```python
from build123d import *

# Parameters (mm, degrees)
ESQUISSE1_R             = 1.5
BOSS_EXTRU_1_DEPTH      = 10.4
ESQUISSE2_R             = 1.5
BOSS_EXTRU_3_DEPTH      = 0.2
BOSS_EXTRU_4_START      = 0.2
ESQUISSE3_R             = 1.5
BOSS_EXTRU_4_DEPTH      = 0.2
ENL_V_MAT_EXTRU_1_DEPTH = 0.2
ENL_V_MAT_EXTRU_3_DEPTH = 0.5
ENL_V_MAT_EXTRU_4_DEPTH = 0.5
CONG_1_R                = 0.4
ESQUISSE8_R             = 2
BOSS_EXTRU_5_DEPTH      = 3
CONG_2_R                = 0.4
ESQUISSE9_W             = 7
ESQUISSE9_H             = 12.59732845
ESQUISSE9_R             = 1.25
ENL_V_MAT_EXTRU_5_DEPTH = 0.1
BOSS_EXTRU_6_START      = 0.75
BOSS_EXTRU_6_DEPTH      = 0.75
BOSS_EXTRU_7_START      = 1
BOSS_EXTRU_7_DEPTH      = 1
CONG_3_R                = 1


with BuildPart() as part:
    # Esquisse1 → Boss.-Extru.1 (new body)
    with BuildSketch(Plane(origin=(0, 0, 0), x_dir=(0, 0, -1), z_dir=(1, 0, 0))):
        with BuildLine():
            Line((2.8, 0), (15, 0))
            Line((15, 0), (20, 5))
            Line((20, 5), (20, 31))
            Line((20, 31), (2.8, 31))
            ThreePointArc((2.8, 31), (0.820101013, 30.179898987), (0, 28.2))
            Line((0, 28.2), (0, 2.8))
            ThreePointArc((0, 2.8), (0.820101013, 0.820101013), (2.8, 0))
        make_face()
        with Locations((3, 28.2)):
            Circle(ESQUISSE1_R, mode=Mode.SUBTRACT)
        with Locations((3, 2.8)):
            Circle(ESQUISSE1_R, mode=Mode.SUBTRACT)
    extrude(amount=BOSS_EXTRU_1_DEPTH)

    # Esquisse2 → Boss.-Extru.3 (add)
    with BuildSketch(Plane(origin=(10.4, 0, 0), x_dir=(0, 0, -1), z_dir=(1, 0, 0))):
        with BuildLine():
            Line((5.15, 28.2), (5.15, 2.8))
            ThreePointArc((5.15, 2.8), (3, 0.65), (0.85, 2.8))
            Line((0.85, 2.8), (0.85, 28.2))
            ThreePointArc((0.85, 28.2), (3, 30.35), (5.15, 28.2))
        make_face()
        with Locations((3, 28.2)):
            Circle(ESQUISSE2_R, mode=Mode.SUBTRACT)
        with Locations((3, 2.8)):
            Circle(ESQUISSE2_R, mode=Mode.SUBTRACT)
    extrude(amount=BOSS_EXTRU_3_DEPTH)

    # Esquisse3 → Boss.-Extru.4 (add)
    with BuildSketch(Plane.ZY.offset(BOSS_EXTRU_4_START)):
        with BuildLine():
            Line((-0.85, 28.2), (-0.85, 2.8))
            ThreePointArc((-0.85, 2.8), (-3, 0.65), (-5.15, 2.8))
            Line((-5.15, 2.8), (-5.15, 28.2))
            ThreePointArc((-5.15, 28.2), (-3, 30.35), (-0.85, 28.2))
        make_face()
        with Locations((-3, 2.8)):
            Circle(ESQUISSE3_R, mode=Mode.SUBTRACT)
        with Locations((-3, 28.2)):
            Circle(ESQUISSE3_R, mode=Mode.SUBTRACT)
    extrude(amount=-BOSS_EXTRU_4_DEPTH)

    # Esquisse4 → Enlèv. mat.-Extru.1 (cut)
    with BuildSketch(Plane.XY):
        with BuildLine():
            Line((2.2, 24.5), (8.2, 24.5))
            ThreePointArc((8.2, 24.5), (8.907106781, 24.207106781), (9.2, 23.5))
            Line((9.2, 23.5), (9.2, 7.5))
            ThreePointArc((9.2, 7.5), (8.907106781, 6.792893219), (8.2, 6.5))
            Line((8.2, 6.5), (2.2, 6.5))
            ThreePointArc((2.2, 6.5), (1.492893219, 6.792893219), (1.2, 7.5))
            Line((1.2, 7.5), (1.2, 23.5))
            ThreePointArc((1.2, 23.5), (1.492893219, 24.207106781), (2.2, 24.5))
        make_face()
        with BuildLine():
            Line((8.7, 19.5), (8.7, 11.5))
            ThreePointArc((8.7, 11.5), (5.2, 8), (1.7, 11.5))
            Line((1.7, 11.5), (1.7, 19.5))
            ThreePointArc((1.7, 19.5), (5.2, 23), (8.7, 19.5))
        make_face(mode=Mode.SUBTRACT)
    extrude(amount=-ENL_V_MAT_EXTRU_1_DEPTH, mode=Mode.SUBTRACT)

    # Esquisse5 → Enlèv. mat.-Extru.3 (cut)
    with BuildSketch(Plane(origin=(10.4, 0, 0), x_dir=(0, 0, -1), z_dir=(1, 0, 0))):
        Polygon((13, 0), (20, 7), (20, 7.707106781), (12.292893219, 0), align=None)
        Polygon((11.585786438, 0), (20, 8.414213562), (20, 9.121320344), (10.878679656, 0), align=None)
        Polygon((20, 9.828427125), (10.171572875, 0), (9.464466094, 0), (20, 10.535533906), align=None)
        Polygon((20, 11.242640687), (8.757359313, 0), (8.050252532, 0), (20, 11.949747468), align=None)
        Polygon((7.343145751, 0), (20, 12.656854249), (20, 13.363961031), (6.636038969, 0), align=None)
    extrude(amount=-ENL_V_MAT_EXTRU_3_DEPTH, mode=Mode.SUBTRACT)

    # Esquisse7 → Enlèv. mat.-Extru.4 (cut)
    with BuildSketch(Plane.ZY):
        Polygon((-20, 7), (-13, 0), (-12.292893219, 0), (-20, 7.707106781), align=None)
        Polygon((-20, 8.414213562), (-11.585786438, 0), (-10.878679656, 0), (-20, 9.121320344), align=None)
        Polygon((-20, 9.828427125), (-20, 10.535533906), (-9.464466094, 0), (-10.171572875, 0), align=None)
        Polygon((-20, 11.242640687), (-8.757359313, 0), (-8.050252532, 0), (-20, 11.949747468), align=None)
        Polygon((-20, 12.656854249), (-20, 13.363961031), (-6.636038969, 0), (-7.343145751, 0), align=None)
    extrude(amount=-ENL_V_MAT_EXTRU_4_DEPTH, mode=Mode.SUBTRACT)

    # Congé1
    cong_1_edges = [part.edges().sort_by_distance(p)[0] for p in [
        (10.4, 30.179898987, -0.820101013),
        (5.2, 5, -20),
        (5.2, 0, -15),
        (5.2, 31, -20),
        (10.4, 15.5, 0),
        (10.4, 22.181980515, -20),
        (10.4, 0.820101013, -0.820101013),
        (0, 0, -14),
        (10.4, 0, -4.718019485),
        (10.4, 2.5, -17.5),
        (0, 22.181980515, -20),
        (10.4, 6, -20),
        (0, 2.5, -17.5),
        (10.4, 31, -11.4),
        (0, 0, -4.718019485),
        (0, 0.820101013, -0.820101013),
        (0, 15.5, 0),
        (0, 30.179898987, -0.820101013),
        (0, 31, -11.4),
        (0, 6, -20),
        (10.4, 0, -14),
    ]]
    fillet(cong_1_edges, radius=CONG_1_R)

    # Esquisse8 → Boss.-Extru.5 (add)
    with BuildSketch(Plane(origin=(0, -7.5, -7.5), x_dir=(1, 0, 0), z_dir=(0, -0.7071067811865512, -0.7071067811865438))):
        with Locations(Location((5.2, -14.142135624, 0), (0, 0, 90))):
            Circle(ESQUISSE8_R)
    extrude(amount=BOSS_EXTRU_5_DEPTH)

    # Congé2
    cong_2_edges = [part.edges().sort_by_distance(p)[0] for p in [
        (5.2, 3.914213562, -18.914213562),
    ]]
    fillet(cong_2_edges, radius=CONG_2_R)

    # Esquisse9 → Enlèv. mat.-Extru.5 (cut)
    with BuildSketch(Plane(origin=(0, 31, 0), x_dir=(1, 0, 0), z_dir=(0, 1, 0))):
        with Locations((5.2, 11.2)):
            Rectangle(ESQUISSE9_W, ESQUISSE9_H)
        with Locations(Location((5.2, 15.836199023, 0), (0, 0, 270))):
            Circle(ESQUISSE9_R, mode=Mode.SUBTRACT)
        with Locations(Location((5.2, 11.836199023, 0), (0, 0, 270))):
            Circle(ESQUISSE9_R, mode=Mode.SUBTRACT)
        with BuildLine():
            Line((3.6, 6.378161231), (6.8, 6.378161231))
            ThreePointArc((6.8, 6.378161231), (8.245782033, 8.277803961), (6.029604961, 9.165208815))
            ThreePointArc((6.029604961, 9.165208815), (5.2, 8.935889606), (4.370395039, 9.165208815))
            ThreePointArc((4.370395039, 9.165208815), (2.154217967, 8.277803961), (3.6, 6.378161231))
        make_face(mode=Mode.SUBTRACT)
    extrude(amount=-ENL_V_MAT_EXTRU_5_DEPTH, mode=Mode.SUBTRACT)

    # Esquisse10 → Boss.-Extru.6 (add)
    with BuildSketch(Plane(origin=(0, 31, 0), x_dir=(1, 0, 0), z_dir=(0, 1, 0)).offset(BOSS_EXTRU_6_START)):
        with BuildLine():
            Line((3.954711438, 15.727772098), (6.159077004, 16.637866847))
            ThreePointArc((6.159077004, 16.637866847), (4.722980738, 16.991600522), (3.954711438, 15.727772098))
        make_face()
        with BuildLine():
            Line((4.240922996, 15.034531199), (6.445288562, 15.944625947))
            ThreePointArc((6.445288562, 15.944625947), (5.677019262, 14.680797524), (4.240922996, 15.034531199))
        make_face()
        with BuildLine():
            Line((4.042878005, 11.363368516), (5.878209102, 12.886214458))
            ThreePointArc((5.878209102, 12.886214458), (4.401811845, 12.798173903), (4.042878005, 11.363368516))
        make_face()
        with BuildLine():
            Line((4.521790898, 10.786183588), (6.357121995, 12.30902953))
            ThreePointArc((6.357121995, 12.30902953), (5.998188155, 10.874224143), (4.521790898, 10.786183588))
        make_face()
    extrude(amount=-BOSS_EXTRU_6_DEPTH)

    # Esquisse12 → Boss.-Extru.7 (add)
    with BuildSketch(Plane(origin=(0, 31, 0), x_dir=(1, 0, 0), z_dir=(0, 1, 0)).offset(BOSS_EXTRU_7_START)):
        with BuildLine():
            Line((3.6, 6.378161231), (6.8, 6.378161231))
            ThreePointArc((6.8, 6.378161231), (8.245782033, 8.277803961), (6.029604961, 9.165208815))
            ThreePointArc((6.029604961, 9.165208815), (5.2, 8.935889606), (4.370395039, 9.165208815))
            ThreePointArc((4.370395039, 9.165208815), (2.154217967, 8.277803961), (3.6, 6.378161231))
        make_face()
    extrude(amount=-BOSS_EXTRU_7_DEPTH)

    # Congé3
    cong_3_edges = [part.edges().sort_by_distance(p)[0] for p in [
        (5.2, 32, -8.935889606),
        (2.154217967, 32, -8.277803961),
        (5.2, 32, -6.378161231),
        (8.245782033, 32, -8.277803961),
    ]]
    fillet(cong_3_edges, radius=CONG_3_R - 0.0001)  # a hair under: the kernel refuses the full size


solid = part.part
```
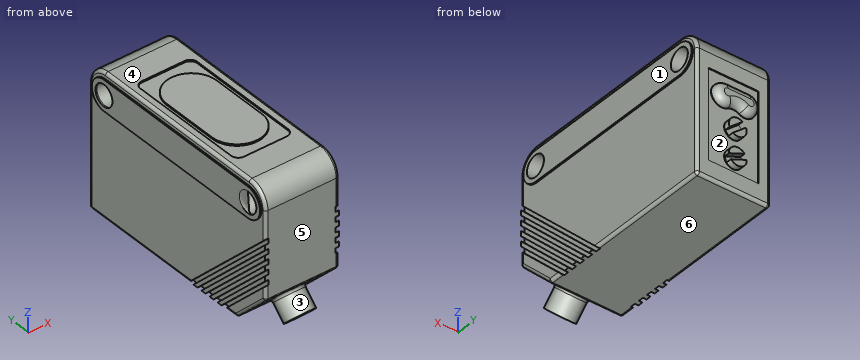
CAD build for the part. Positions are in the model's coordinates, mm. Face numbers are marked on the shaded views. A direction names the side the tool comes from. Round coordinates to 2 decimals unless told otherwise and drop trailing zeros. Write each loop counter-clockwise with the first axis right and the second up, starting at its lowest first coordinate (ties: lowest second). Pieces come first, ordered by that corner, then holes. Notation, with made-up numbers: (41.5, 28) -> (100.5, 28) arc R20 cw to (100.5, 65) -> close; hole circle Ø2 at (-37.75, 9). An arc over 180 degrees is marked (long way). Answer in a Markdown table with one row per item. Add a question column.
Item 1: Mould opens along Y. For the marked faces 1, 2 and 3 say: pulls with the +Y half, pulls with the -Y half, needs draft (parallel to the pull), parting line crosses it, or undercut.
Item 2: Saw through at A-A, the plane y = 19. Write the cut outline in (x, z).
Item 3: Drill centre lines: line 1 (Y direction, x = 4.25, z = -3); line 2 (Z direction, x = 4.25, y = 28.2); line 3 (Y direction, x = 10.25, z = -13.75). Where is each one in solid material? Low to high. Write a range as from..to.
Item 4: Saw through at B-B, the plane x = 5.2. Count the separate pieces of the cut face and the enclosed holes in it, then the cut area to 3 significant figures.
Item 5: Saw through at C-C, the plane y = 24. Write the cut outline in (x, z).
Item 6: Which spindle directions (+Z, -Z, +X, -X, +Y, -Y) get a long thin tool onto all of the face, cutting with end or side? Do the marked faces 4, 5 and 6. Say none if no direction does.
Item 7: Drop flat-ended pins along their axis: pin 1 Ø1.8 at (y, z) = (28.2, -3) entering from +X; pin 2 Ø1.4 at (x, z) = (5, -12) entering from +Y; pin 3 Ø6 at (x, y) = (4, 16) entering from +Z; pin 4 Ø8 at (y, z) = (22, -12) entering from -X. Give the stop position or say it passes through.
Findings below:
| question | item | result |
|---|---|---|
| 1 | face 1 | needs draft |
| 1 | face 2 | pulls with the +Y half |
| 1 | face 3 | undercut |
| 2 | outline | (-0.2, -5.15) -> (0, -5.15) -> (0, -19.6) arc R0.4 ccw to (0.4, -20) -> (10, -20) arc R0.4 ccw to (10.4, -19.6) -> (10.4, -5.15) -> (10.6, -5.15) -> (10.6, -0.85) -> (10.4, -0.85) -> (10.4, -0.4) arc R0.4 ccw to (10, 0) -> (9.2, 0) -> (9.2, -0.2) -> (8.7, -0.2) -> (8.7, 0) -> (1.7, 0) -> (1.7, -0.2) -> (1.2, -0.2) -> (1.2, 0) -> (0.4, 0) arc R0.4 ccw to (0, -0.4) -> (0, -0.85) -> (-0.2, -0.85) -> close |
| 3 | line 1 | y = 0..1.3, 4.3..26.7, 29.7..31 |
| 3 | line 2 | z = -20..-4.5, -1.5..0 |
| 3 | line 3 | y = 0.09..0.75, 1.46..2.16, 2.87..3.58, 4.29..4.99, 5.7..6.41, 7.11..30.91 |
| 4 | separate pieces | 1 |
| 4 | enclosed holes | 2 |
| 4 | area | 605 mm^2 |
| 5 | outline | (-0.2, -5.15) -> (0, -5.15) -> (0, -19.6) arc R0.4 ccw to (0.4, -20) -> (10, -20) arc R0.4 ccw to (10.4, -19.6) -> (10.4, -5.15) -> (10.6, -5.15) -> (10.6, -0.85) -> (10.4, -0.85) -> (10.4, -0.4) arc R0.4 ccw to (10, 0) -> (9.07, 0) -> (9.07, -0.2) -> (1.33, -0.2) -> (1.33, 0) -> (0.4, 0) arc R0.4 ccw to (0, -0.4) -> (0, -0.85) -> (-0.2, -0.85) -> close |
| 6 | face 4 | +Z, +X, -X, +Y, -Y |
| 6 | face 5 | +Z, +X, -X, -Y |
| 6 | face 6 | -Z, +X, -X, +Y |
| 7 | pin 1 | passes through |
| 7 | pin 2 | stops at y = 31.75 |
| 7 | pin 3 | stops at z = 0 |
| 7 | pin 4 | stops at x = 0 |
